Here's how the part is built. I have some questions about the finished solid (model axes, mm). Face numbers are marked on the shaded views. A direction names the side the tool comes from. Round coordinates to 2 decimals unless told otherwise and drop trailing zeros. Loops run counter-clockwise (first coordinate to the right, second up) from the corner with the lowest first, then second, coordinate; pieces in that order, holes last. Notation, with made-up numbers: M -4,10.25 L 16,10.25 A19 ccw 16,25.25 Z; hole C 28.5,70.5 d4. An arc over 180 degrees is marked long. Use a Markdown table: item, result.
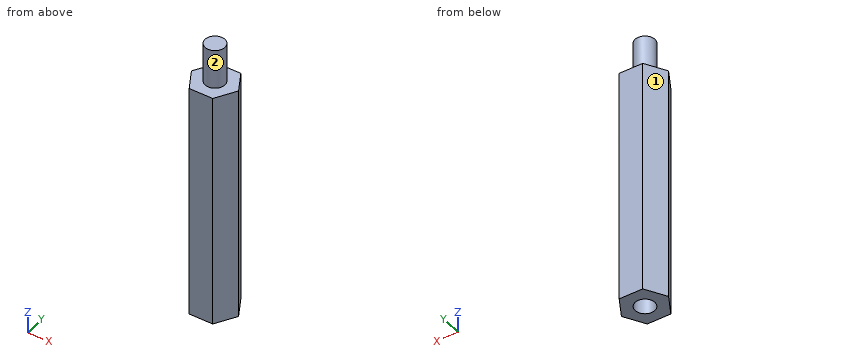
from build123d import *

# Parameters (mm, degrees)
F0_R     = 1.25
F1_DEPTH = 30
F2_DEPTH = 35
F3_R     = 1.25
F4_DEPTH = 28


# Not quite as in the source:
# - a feature names something its author has since deleted; it is built from what else it names


with BuildPart() as f1:
    # F0 (on Top) → F1 (new body)
    with BuildSketch(Plane.XY):
        Polygon((1.5, 2.5980762114), (-1.5, 2.5980762114), (-3, 0), (-1.5, -2.5980762114), (1.5, -2.5980762114), (3, 0), align=None)
        Circle(F0_R, mode=Mode.SUBTRACT)
    extrude(amount=F1_DEPTH)

    # F0 (on Top) → F2 (join)
    with BuildSketch(Plane.XY):
        Circle(F0_R)
    extrude(amount=F2_DEPTH)

    # F3 (on face) → F4 (cut)
    with BuildSketch(Plane(origin=(0, 0, 0), x_dir=(1, 0, 0), z_dir=(0, 0, -1))):
        Circle(F3_R)
    extrude(amount=-F4_DEPTH, mode=Mode.SUBTRACT)


solid = f1.part
1. Imagine slicing it at A-A, the plane z = 16. Write out the boundary of the cut face in (x, y), then the cut area to 3 significant figures.
Answer sheet:
| item | result |
|---|---|
| outline | M -3,0 L -1.5,-2.6 L 1.5,-2.6 L 3,0 L 1.5,2.6 L -1.5,2.6 Z; hole C 0,0 d2.5 |
| area | 18.5 mm2 |
2. For pin 1 Ø1.5 at (y, z) = (0.5, 17.5) entering from +X; pin 2 Ø1.2 at (x, y) = (-0.5, 0) entering from -Z; pin 3 Ø1.5 at (x, z) = (-2.5, 21) entering from -Y, each with a flat end and sliding along its axis, tell me the tip position at first contact or that it passes through.
Answer sheet:
| item | result |
|---|---|
| pin 1 | x = 3 |
| pin 2 | z = 28 |
| pin 3 | y = -2.17 |
3. Imagine slicing it at D-D, the plane y = -2.25. Write out the boundary of the cut face in (x, z).
Answer sheet:
| item | result |
|---|---|
| outline | M -1.7,0 L 1.7,0 L 1.7,30 L -1.7,30 Z |
4. Imagine slicing it at B-B, the plane x = 0. Write out the boundary of the cut face in (y, z), then the cut area to 3 significant figures.
Answer sheet:
| item | result |
|---|---|
| outline | M -2.6,0 L -1.25,0 L -1.25,28 L 1.25,28 L 1.25,0 L 2.6,0 L 2.6,30 L 1.25,30 L 1.25,35 L -1.25,35 L -1.25,30 L -2.6,30 Z |
| area | 98.4 mm2 |
5. I need wall thicknesses on probe 1 along Y at (x, z) = (0, 18); probe 2 along Z at (x, y) = (0.75, 1.1); probe 3 along X at (y, z) = (1.1, 5). Which ranges of each line are inside material? Lowest first, please. Write a range as from..to.
Answer sheet:
| item | result |
|---|---|
| probe 1 | -2.6..-1.25, 1.25..2.6 |
| probe 2 | 0..30 |
| probe 3 | -2.36..-0.59, 0.59..2.36 |
6. Imagine slicing it at C-C, the plane z = 29.5. Write out the boundary of the cut face in (x, y).
Answer sheet:
| item | result |
|---|---|
| outline | M -3,0 L -1.5,-2.6 L 1.5,-2.6 L 3,0 L 1.5,2.6 L -1.5,2.6 Z |
7. Which directions (+Z, -Z, +X, -X, +Y, -Y) give clear straight access to the entire face, cutting with the end or side of a thin tool? Please do the marked faces 1 and 2.
Answer sheet:
| item | result |
|---|---|
| face 1 | +Z, -Z, -X, +Y |
| face 2 | +Z |
